Part model, mm, in its own coordinate system. A direction names the side the tool comes from. Round coordinates to 2 decimals unless told otherwise and drop trailing zeros. Order: outer loops, then holes, each group sorted by start corner. A loop starts at its lowest first (then second) coordinate and runs counter-clockwise, first axis right, second up. Notation, with made-up numbers: (44.25, 11.5) - (62.25, 11.5) arc R28 cw to (62.25, 35.5) - close; hole circle Ø11 at (72.25, 77). An arc over 180 degrees is marked (long way). Answer as a JSON object with one key per item and string values.
```python
from build123d import *

# Parameters (mm, degrees)
SKETCH1_W           = 28
SKETCH1_H           = 63
SKETCH1_W_2         = 20
SKETCH1_H_2         = 41
BOSS_EXTRUDE1_DEPTH = 10.9
SKETCH2_R           = 2
CUT_EXTRUDE1_DEPTH  = 45.904036567
CHAMFER1_SIZE       = 10.9
CHAMFER1_SIZE_2     = 3
SKETCH3_W           = 2
SKETCH3_H           = 1
CUT_EXTRUDE2_DEPTH  = 65.248521384
FILLET1_R           = 2.5


with BuildPart() as part:
    # Sketch1 → Boss-Extrude1 (new body)
    with BuildSketch(Plane.XY):
        with Locations((0, 9.75)):
            Rectangle(SKETCH1_W, SKETCH1_H)
        with Locations((0, 9.75)):
            Rectangle(SKETCH1_W_2, SKETCH1_H_2, mode=Mode.SUBTRACT)
    extrude(amount=BOSS_EXTRUDE1_DEPTH)

    # Sketch2 → Cut-Extrude1 (cut, through all)
    with BuildSketch(Plane(origin=(0, 0, 0), x_dir=(-1, 0, 0), z_dir=(0, 0, -1))):
        with Locations((5.013249621, -14.95)):
            Circle(SKETCH2_R)
        with Locations((-4.986750379, -14.95)):
            Circle(SKETCH2_R)
        with Locations((-5.030525248, 34.45)):
            Circle(SKETCH2_R)
        with Locations((4.969474752, 34.45)):
            Circle(SKETCH2_R)
    extrude(amount=-CUT_EXTRUDE1_DEPTH, mode=Mode.SUBTRACT)

    # Chamfer1
    # the kernel refuses this chamfer: 10.9, 3 mm, written as the material it takes off along each edge
    with BuildSketch(Plane(origin=(14, -50.052400278, 10.9), x_dir=(0.010219792224504668, 0, -0.9999477765598), z_dir=(0, 1, 0)), Plane(origin=(-14, 69.552400278, 10.9), x_dir=(-0.010219792224504668, 0, -0.9999477765598), z_dir=(0, -1, 0))) as chamfer1_piece_1:
        Polygon((CHAMFER1_SIZE * 0.99994777656, CHAMFER1_SIZE * 0.0102197922245), (-CHAMFER1_SIZE_2 * 0.0102197922245, CHAMFER1_SIZE_2 * 0.99994777656), (0, 0), align=None)
    extrude(amount=119.604800556, mode=Mode.SUBTRACT)
    with BuildSketch(Plane(origin=(-42.302400278, -21.75, 10.9), x_dir=(0, -0.010219792224504825, -0.9999477765598), z_dir=(1, 0, 0))) as chamfer1_piece_2:
        Polygon((CHAMFER1_SIZE * 0.99994777656, CHAMFER1_SIZE * 0.0102197922245), (-CHAMFER1_SIZE_2 * 0.0102197922245, CHAMFER1_SIZE_2 * 0.99994777656), (0, 0), align=None)
    extrude(amount=84.604800556, mode=Mode.SUBTRACT)
    with BuildSketch(Plane(origin=(42.302400278, 41.25, 10.9), x_dir=(0, -0.9910207476808653, 0.1337081809989902), z_dir=(-1, 0, 0))) as chamfer1_piece_3:
        Polygon((CHAMFER1_SIZE_2 * 0.991020747681, -CHAMFER1_SIZE_2 * 0.133708180999), (-CHAMFER1_SIZE * 0.133708180999, -CHAMFER1_SIZE * 0.991020747681), (0, 0), align=None)
    extrude(amount=84.604800556, mode=Mode.SUBTRACT)

    # Sketch3 → Cut-Extrude2 (cut, through all)
    with BuildSketch(Plane(origin=(0, 40, 0), x_dir=(1, 0, 0), z_dir=(0, 1, 0))):
        with Locations((0, -10.4)):
            Rectangle(SKETCH3_W, SKETCH3_H)
    extrude(amount=-CUT_EXTRUDE2_DEPTH, mode=Mode.SUBTRACT)

    # Fillet1
    fillet1_edges = [part.edges().sort_by_distance(p)[0] for p in [
        (-12.5, -20.25, 5.45),
        (-12.5, 39.75, 5.45),
        (12.5, -20.25, 5.45),
        (12.5, 39.75, 5.45),
    ]]
    fillet(fillet1_edges, radius=FILLET1_R)


solid = part.part
```
Item 1: Cut at A-A (x = 0). Write the cut outline in (y, z).
Taken from the geometry:
{"outline": "(-21.75, 0) - (-10.75, 0) - (-10.75, 9.9) - (-19.03, 9.9) - close; (30.25, 0) - (41.25, 0) - (38.53, 9.9) - (30.25, 9.9) - close"}
Item 2: Drop flat-ended pins along their axis: P1, Ø3, axis at x = 5.03, y = 34.45, coming from the +Z side; P2, Ø0.8, axis at y = -16, z = 10.5, coming from the +X side; P3, Ø1.1, axis at y = 34, z = 10.5, coming from the +X side; P4, Ø2, axis at y = 27, z = 4.5, coming from the -X side. Give the stop position or say it passes through.
Taken from the geometry:
{"P1": "through", "P2": "x = 11.22", "P3": "x = 11.26", "P4": "x = -13.04"}
Item 3: Tool access for faces 4 (the cylindrical face through (11.787, -19.574, 5.445)), 5 (the flat face through (10, 9, 5)), 6 (the flat face through (0, -15, 9.9)): list every direction of +Z, -Z, +X, -X, +Y, -Y with a clear straight run to the whole face (end or side of a thin tool).
Taken from the geometry:
{"face 4": "+Z, +X, -Y", "face 5": "+Z, -Z", "face 6": "+Z, +Y, -Y"}
Item 4: Cut at D-D (x = -5.5). Write the cut outline in (y, z), plus the area to 3 significant figures.
Taken from the geometry:
{"outline": "(-21.75, 0) - (-16.89, 0) - (-16.89, 10.9) - (-18.75, 10.9) - close; (-13.01, 0) - (-10.75, 0) - (-10.75, 10.9) - (-13.01, 10.9) - close; (30.25, 0) - (32.52, 0) - (32.52, 10.9) - (30.25, 10.9) - close; (36.38, 0) - (41.25, 0) - (38.25, 10.9) - (36.38, 10.9) - close", "area": "123 mm2"}
Item 5: Cut at B-B (y = 14). Write the cut outline in (x, z).
Taken from the geometry:
{"outline": "(-14, 0) - (-10, 0) - (-10, 10.9) - (-11, 10.9) - close; (10, 0) - (14, 0) - (11, 10.9) - (10, 10.9) - close"}
Item 6: Cut at C-C (y = -14.95). Write the cut outline in (x, z).
Taken from the geometry:
{"outline": "(-14, 0) - (-7.01, 0) - (-7.01, 10.9) - (-11, 10.9) - close; (-3.01, 0) - (2.99, 0) - (2.99, 10.9) - (1, 10.9) - (1, 9.9) - (-1, 9.9) - (-1, 10.9) - (-3.01, 10.9) - close; (6.99, 0) - (14, 0) - (11, 10.9) - (6.99, 10.9) - close"}
Item 7: Probe L1, parallel to Y at x = -6.25, z = 2.25; L2, parallel to Y at x = 5.25, z = 4.25; L3, parallel to X at y = 35.5, z = 6.75. List the from-to ranges inside material, lowest first. Write a range as from..to.
Taken from the geometry:
{"L1": "-21.13..-16.52, -13.38..-10.75, 30.25..32.91, 35.99..40.63", "L2": "-20.58..-16.93, -12.97..-10.75, 30.25..32.46, 36.44..40.08", "L3": "-12.14..-6.67, -3.27..3.33, 6.73..12.14"}
Item 8: Two-plate mould, pull along Y, no slides. Class faces 1 (the cylindrical face through (-4.58, -16.902, 5.374)), 2 (the cylindrical face through (-11.781, -19.493, 5.602)), 3 (the flat face through (-12.52, 10.16, 5.37)): pulls with the +Y half, pulls with the -Y half, needs draft (parallel to the pull), parting line crosses it, or undercut.
Taken from the geometry:
{"face 1": "undercut", "face 2": "pulls with the -Y half", "face 3": "needs draft"}
